from build123d import *

# Parameters (mm, degrees)
SKETCH_1_R               = 8.5
EXTRUDE_1_DEPTH          = 4
SKETCH_2_R               = 1.6
CUT_EXTRUDE_1_DEPTH      = 10
CUT_EXTRUDE_3_DEPTH      = 1
CUT_EXTRUDE_3_DEPTH_BACK = 4


with BuildPart() as part:
    # 草图1 → 凸台-拉伸1 (new body)
    with BuildSketch(Plane.XY):
        with BuildLine():
            ThreePointArc((-14.058374697, -11.241089844), (0, -18), (14.058374697, -11.241089844))
            ThreePointArc((14.058374697, -11.241089844), (16.887495374, -9.75), (16.76425672, -6.554364701))
            ThreePointArc((16.76425672, -6.554364701), (15.588457268, 9), (2.705882023, 17.795454545))
            ThreePointArc((2.705882023, 17.795454545), (0, 19.5), (-2.705882023, 17.795454545))
            ThreePointArc((-2.705882023, 17.795454545), (-15.588457268, 9), (-16.76425672, -6.554364701))
            ThreePointArc((-16.76425672, -6.554364701), (-16.887495374, -9.75), (-14.058374697, -11.241089844))
        make_face()
        Circle(SKETCH_1_R, mode=Mode.SUBTRACT)
    extrude(amount=EXTRUDE_1_DEPTH)

    # 草图2 → 切除-拉伸1 (cut)
    with BuildSketch(Plane.XY.offset(4)):
        with Locations((0, 17)):
            Circle(SKETCH_2_R)
        with Locations((14.722431864, -8.5)):
            Circle(SKETCH_2_R)
        with Locations((-14.722431864, -8.5)):
            Circle(SKETCH_2_R)
    extrude(amount=-CUT_EXTRUDE_1_DEPTH, mode=Mode.SUBTRACT)

    # 草图3 → 切除-拉伸3 (cut, two sides)
    with BuildSketch(Plane(origin=(0, 0, 0), x_dir=(-1, 0, 0), z_dir=(0, 0, -1))) as cut_extrude_3_sk:
        with BuildLine():
            ThreePointArc((-0.5, 8.485281374), (0, 8.5), (0.5, 8.485281374))
            Line((0.5, 8.485281374), (0.5, 11))
            Line((0.5, 11), (-0.5, 11))
            Line((-0.5, 11), (-0.5, 8.485281374))
        make_face()
    extrude(amount=CUT_EXTRUDE_3_DEPTH, mode=Mode.SUBTRACT)
    extrude(cut_extrude_3_sk.sketch, amount=-CUT_EXTRUDE_3_DEPTH_BACK, mode=Mode.SUBTRACT)


solid = part.part
The listing builds one solid part. Answer for the finished solid, in the listing's coordinates (mm). A direction names the side the tool comes from. Coordinates: 2 decimals unless noted, no trailing zeros. Order: outer loops, then holes, each group sorted by start corner. A loop starts at its lowest first (then second) coordinate and runs counter-clockwise, first axis right, second up.
Q1. For a pull along Y with two mould halves and no side action, classify faces 1 (the face through (0, 19.5, 2)), 2 (the face through (-16.91, -9.71, 1.97)), 3 (the face through (0, -18, 2)) as pulls with the +Y half, pulls with the -Y half, needs draft (parallel to the pull), parting line crosses it, or undercut.
Q2. A cutting plane is placed at D-D, the plane y = -12. Write down the section's boundary in (x, z).
Q3. A cutting plane is placed at B-B, the plane y = 17. Write down the section's boundary in (x, z), and give its area (3 significant figures).
Q4. Given P1, Ø1.5, axis at x = -1.5, z = 3.5, coming from the -Y side; P2, Ø2, axis at x = -9.5, z = 0.5, coming from the -Y side; P3, Ø1.9, axis at x = 14.72, y = -8.5, coming from the +Z side; P4, Ø0.8, axis at y = 9.5, z = 2, coming from the -X side, each flat-ended and moving along its own axis, determine where each tip first touches the part or whether it passes through.
Q5. Consider line 1 (Y direction, x = 0, z = 2.25); line 2 (X direction, y = 0, z = 3.25); line 3 (X direction, y = -2, z = 1.65). Determine where each line is inside the solid, lowest interval first.
Q6. Which of the six approach directions +Z, -Z, +X, -X, +Y, -Y give full straight-line access (tool end or side, diameter ignored) to faces 4 (the face through (-0.5, 10, 2)), 5 (the face through (-8.3, -3.2, 4))?
Q7. A cutting plane is placed at A-A, the plane x = 0. Write down the section's boundary in (y, z), and give its area (3 significant figures).
Q8. A cutting plane is placed at C-C, the plane z = 0.75. Write down the section's boundary in (x, y).
Answers follow:
1. face 1: pulls with the +Y half
1. face 2: undercut
1. face 3: pulls with the -Y half
2. outline: (-13.42, 0) - (13.42, 0) - (13.42, 4) - (-13.42, 4) - close
3. outline: (-5.92, 0) - (-1.6, 0) - (-1.6, 4) - (-5.92, 4) - close; (1.6, 0) - (5.92, 0) - (5.92, 4) - (1.6, 4) - close
3. area: 34.5 mm2
4. P1: stops at y = -17.98
4. P2: stops at y = -15.87
4. P3: passes through
4. P4: stops at x = -15.53
5. line 1: y = -18 to -8.5, 11 to 15.4, 18.6 to 19.5
5. line 2: x = -18 to -8.5, 8.5 to 18
5. line 3: x = -17.89 to -8.26, 8.26 to 17.89
6. face 4: +Z, -Z
6. face 5: +Z, +X, -X, +Y, -Y
7. outline: (-18, 0) - (-8.5, 0) - (-8.5, 4) - (-18, 4) - close; (11, 0) - (15.4, 0) - (15.4, 4) - (11, 4) - close; (18.6, 0) - (19.5, 0) - (19.5, 4) - (18.6, 4) - close
7. area: 59.2 mm2
8. outline: (-16.76, -6.55) arc R3 ccw to (-14.06, -11.24) arc R18 ccw to (14.06, -11.24) arc R3 ccw to (16.76, -6.55) arc R18 ccw to (2.71, 17.8) arc R3 ccw to (-2.71, 17.8) arc R18 ccw to start; hole circle Ø3.2 at (-14.72, -8.5); hole circle Ø3.2 at (0, 17); hole (-0.5, 8.49) arc R8.5 ccw (long way) to (0.5, 8.49) - (0.5, 11) - (-0.5, 11) - close; hole circle Ø3.2 at (14.72, -8.5)
